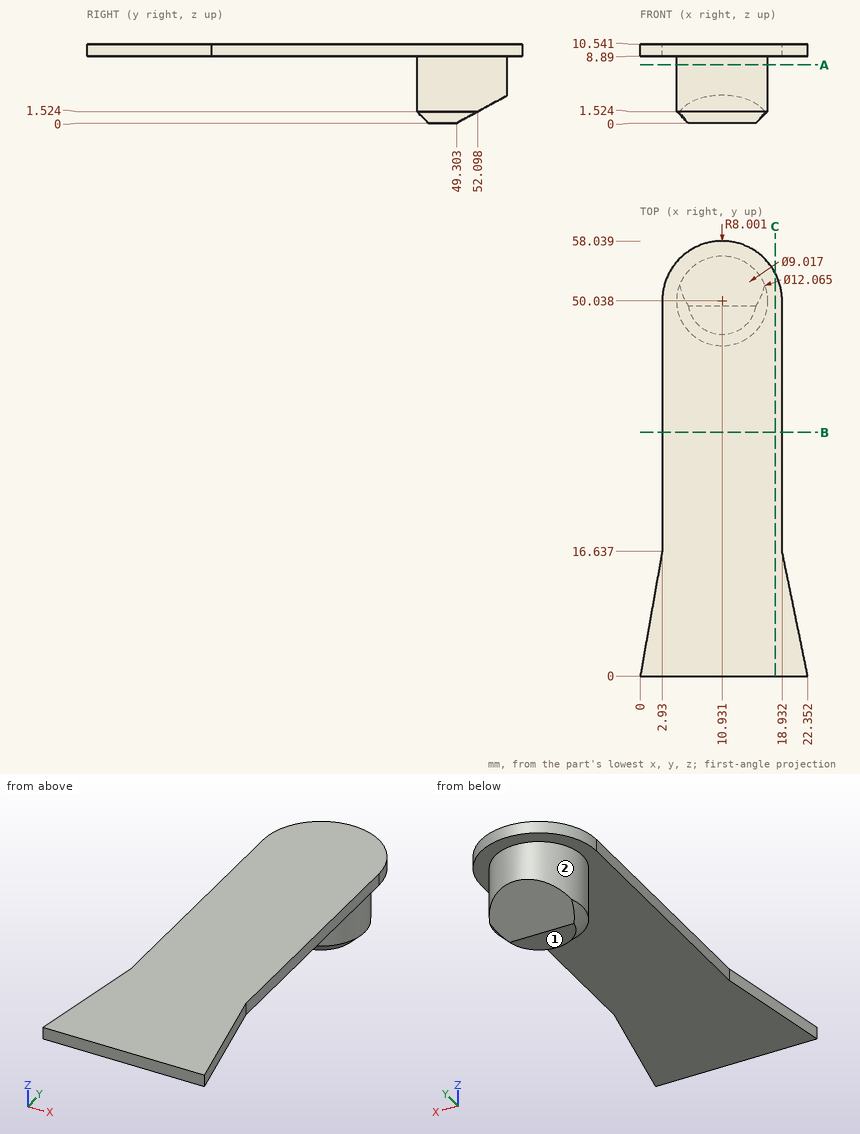
The drawing under review shows one solid part. Ordinate dimensions are in mm from its lowest x, y, z. A direction names the side the tool comes from. Give positions to 0.01 mm unless a question says otherwise; leave off trailing zeros. Order: outer loops, then holes, each group sorted by start corner. A loop starts at its lowest first (then second) coordinate and runs counter-clockwise, first axis right, second up. Notation, with made-up numbers: (-25, 37.5) -> (-14, 37.5) arc R15 ccw to (-14, 58.5) -> close; hole circle Ø7 at (21.5, -9). An arc over 180 degrees is marked (long way). Write item = value, one per line.
1) We need section C-C, the plane x = 18. Give the boundary of the cut face in (y, z).
Findings:
outline = (0, 8.89) -> (53.79, 8.89) -> (53.79, 10.54) -> (0, 10.54) -> close
2) We need section B-B, the plane y = 32.5. Give the boundary of the cut face in (x, z), and give its area (3 significant figures).
Findings:
outline = (2.93, 8.89) -> (18.93, 8.89) -> (18.93, 10.54) -> (2.93, 10.54) -> close
area = 26.4 mm^2
3) Insertion check: pin 1 (2 mm diameter, centred on x = 19, z = 3, fed in from +Y); pin 2 (11 mm diameter, centred on x = 14, y = 39.5, fed in from -Z); pin 3 (0.8 mm diameter, centred on y = 36, z = 9.5, fed in from -X); pin 4 (1.3 mm diameter, centred on y = 35.5, z = 9.5, fed in from +X). Each pin has a flat end and moves straight along its axis. Give the tip position at first contact, or say it passes through.
Findings:
pin_1 = through
pin_2 = 0.97
pin_3 = 2.93
pin_4 = 18.93
4) We need section A-A, the plane z = 7.75. Give the boundary of the cut face in (x, y) (1 decimal), and give its area (3 significant figures).
Findings:
outline = circle Ø12.1 at (10.9, 50)
area = 114 mm^2
5) To check wall thickness, follow L1, parallel to Z at x = 14.5, y = 23; L2, parallel to X at y = 35, z = 10; L3, parallel to Z at x = 11, y = 50.5. State the ranges of each line that lie inside material, in increasing order. Write a range as from..to.
Findings:
L1 = 8.89..10.54
L2 = 2.93..18.93
L3 = 0.65..10.54
6) For the marked faces 1 and 2, list the 3-axis set-ups (+Z, -Z, +X, -X, +Y, -Y) from which the entire face can be reached by the end or side of a thin tool; tool diameter is ignored.
Findings:
face_1 = -Z, +X, -X, +Y, -Y
face_2 = -Z
